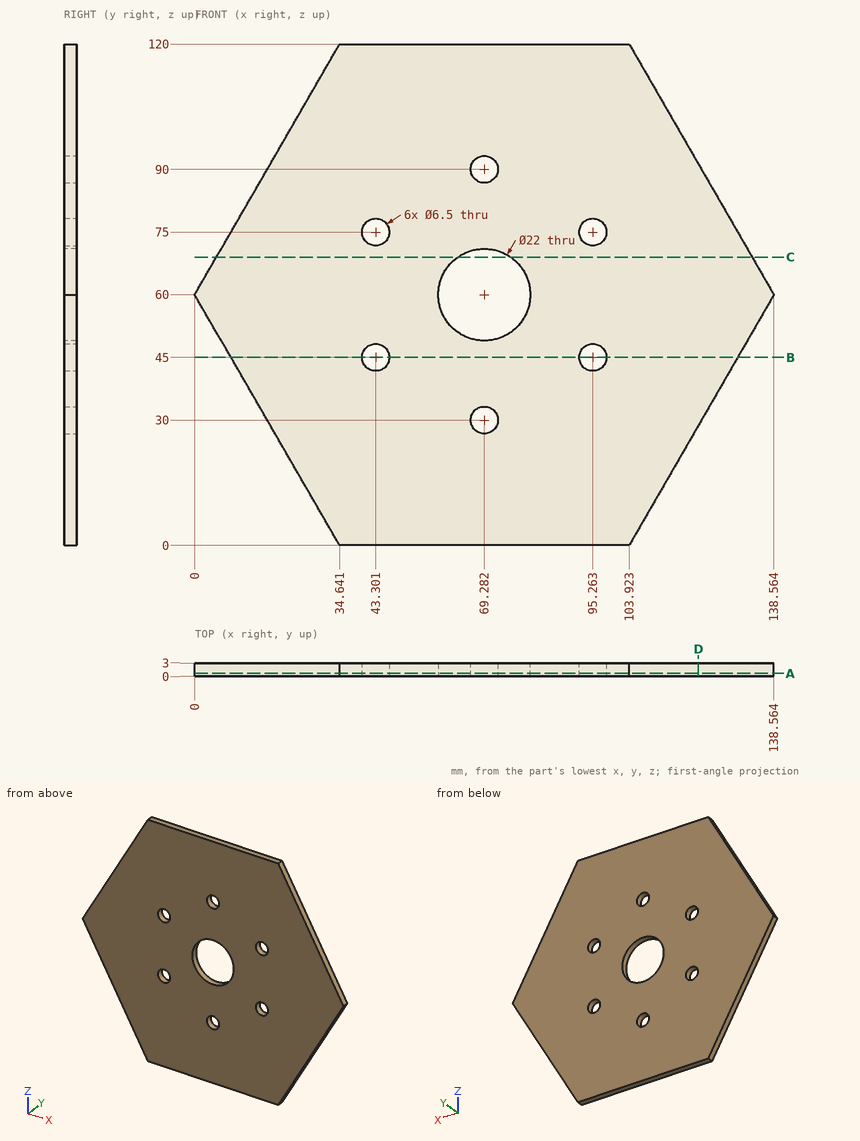
Here's the drawing with two shaded views (mm, measured from the low corner). I have some questions. Coordinates: 2 decimals unless noted, no trailing zeros. Write each loop counter-clockwise with the first axis right and the second up, starting at its lowest first coordinate (ties: lowest second). Pieces come first, ordered by that corner, then holes.
Item 1: I want a section at C-C on z = 69. Write out the boundary of the cut face in (x, y).
Item 2: If I drill on line 1 (X direction, y = 0.7, z = 60) (1 decimal); line 2 (Z direction, x = 94, y = 0.5) (1 decimal); line 3 (X direction, y = 2.35, z = 75), over which ranges is the centre line in solid material (lowest first)?
Item 3: I want a section at B-B on z = 45. Write out the boundary of the cut face in (x, y).
Item 4: Will this pin go through, and if not, where does the flat tip stop? pin 1 (5 mm diameter, centred on x = 43.3, z = 75, fed in from -Y).
Item 5: I want a section at D-D on x = 120.5. Write out the boundary of the cut face in (y, z).
Item 6: I want a section at A-A on y = 0.65. Write out the boundary of the cut face in (x, z).
Findings below:
1. outline: (5.2, 0) - (62.96, 0) - (62.96, 3) - (5.2, 3) - close; (75.61, 0) - (133.37, 0) - (133.37, 3) - (75.61, 3) - close
2. line 1: x = 0 to 58.3, 80.3 to 138.6
2. line 2: z = 0 to 42, 48 to 72, 78 to 120
2. line 3: x = 8.66 to 40.05, 46.55 to 92.01, 98.51 to 129.9
3. outline: (8.66, 0) - (40.05, 0) - (40.05, 3) - (8.66, 3) - close; (46.55, 0) - (92.01, 0) - (92.01, 3) - (46.55, 3) - close; (98.51, 0) - (129.9, 0) - (129.9, 3) - (98.51, 3) - close
4. pin 1: passes through
5. outline: (0, 28.71) - (3, 28.71) - (3, 91.29) - (0, 91.29) - close
6. outline: (0, 60) - (34.64, 0) - (103.92, 0) - (138.56, 60) - (103.92, 120) - (34.64, 120) - close; hole circle Ø6.5 at (43.3, 45); hole circle Ø6.5 at (43.3, 75); hole circle Ø22 at (69.28, 60); hole circle Ø6.5 at (69.28, 30); hole circle Ø6.5 at (69.28, 90); hole circle Ø6.5 at (95.26, 45); hole circle Ø6.5 at (95.26, 75)
